Answer from the drawing. Dimensions are ordinates in mm from the lowest x, y and z of the part. A direction names the side the tool comes from. Round coordinates to 2 decimals unless told otherwise and drop trailing zeros. Write each loop counter-clockwise with the first axis right and the second up, starting at its lowest first coordinate (ties: lowest second). Pieces come first, ordered by that corner, then holes. Notation, with made-up numbers: (45.5, 28) - (88.5, 28) arc R30 cw to (88.5, 62) - close; hole circle Ø9 at (16, -26). An arc over 180 degrees is marked (long way). Answer as a JSON object with one key per item and string values.
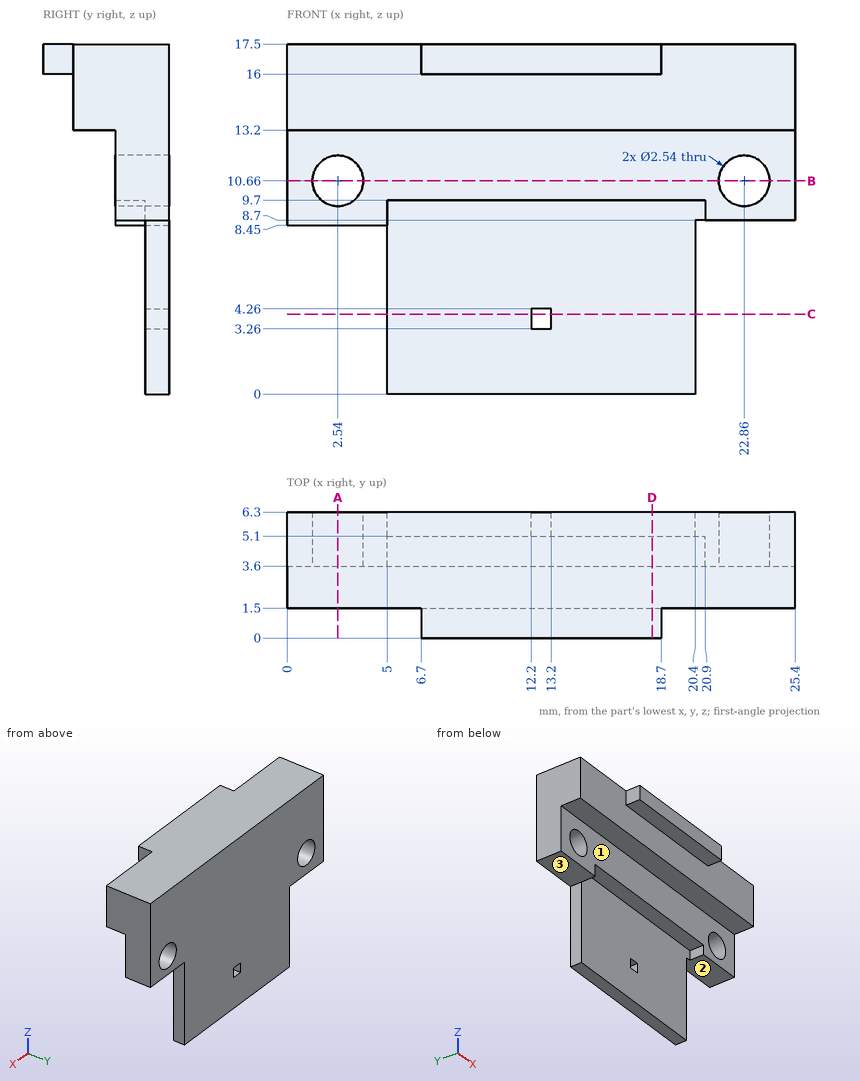
Item 1: A cutting plane is placed at B-B (z = 10.66). Write down the section's boundary in (x, y), and give its area (3 significant figures).
Results found:
{"outline": "(0, 3.6) - (1.27, 3.6) - (1.27, 6.3) - (0, 6.3) - close; (3.81, 3.6) - (21.59, 3.6) - (21.59, 6.3) - (3.81, 6.3) - close; (24.13, 3.6) - (25.4, 3.6) - (25.4, 6.3) - (24.13, 6.3) - close", "area": "54.9 mm²"}
Item 2: Consider line 1 along X through (y, z) = (4.65, 10.66); line 2 along Z through (x, y) = (2.54, 5.45); line 3 along Z through (x, y) = (22.86, 4.55). Determine where each line is inside the solid, lowest interval first.
Results found:
{"line 1": "0 to 1.27, 3.81 to 21.59, 24.13 to 25.4", "line 2": "8.45 to 9.39, 11.93 to 17.5", "line 3": "8.7 to 9.39, 11.93 to 17.5"}
Item 3: A cutting plane is placed at C-C (z = 4). Write down the section's boundary in (x, y).
Results found:
{"outline": "(5, 5.1) - (12.2, 5.1) - (12.2, 6.3) - (5, 6.3) - close; (13.2, 5.1) - (20.4, 5.1) - (20.4, 6.3) - (13.2, 6.3) - close"}
Item 4: For the marked faces 1, 2 and 3, determine the directions among +Z, -Z, +X, -X, +Y, -Y from which every point of the face is accessible in a straight line to the end or side of a thin tool.
Results found:
{"face 1": "-Z, +X, -X, -Y", "face 2": "-Z, +X, +Y, -Y", "face 3": "-Z, -X, +Y, -Y"}
Item 5: Each of these flat-tipped pins is pushed along its axis until it touches: P1, Ø2.5, axis at x = 13.5, z = 11, coming from the -Y side; P2, Ø3, axis at y = 5, z = 4.5, coming from the -X side; P3, Ø1.4, axis at x = 21.5, y = 5, coming from the -Z side. Where does it stop, or does it pass through?
Results found:
{"P1": "y = 3.6", "P2": "x = 5", "P3": "z = 8.7"}
Item 6: A cutting plane is placed at A-A (x = 2.54). Write down the section's boundary in (y, z).
Results found:
{"outline": "(1.5, 13.2) - (3.6, 13.2) - (3.6, 11.93) - (6.3, 11.93) - (6.3, 17.5) - (1.5, 17.5) - close; (3.6, 8.45) - (6.3, 8.45) - (6.3, 9.39) - (3.6, 9.39) - close"}
Item 7: A cutting plane is placed at D-D (x = 18.25). Write down the section's boundary in (y, z), and give its area (3 significant figures).
Results found:
{"outline": "(0, 16) - (1.5, 16) - (1.5, 13.2) - (3.6, 13.2) - (3.6, 9.7) - (5.1, 9.7) - (5.1, 0) - (6.3, 0) - (6.3, 17.5) - (0, 17.5) - close", "area": "44.0 mm²"}
